Geometry: final body of the model. Coordinates: model frame, mm. A direction names the side the tool comes from. Give positions to 0.01 mm unless a question says otherwise; leave off trailing zeros. Loops run counter-clockwise (first coordinate to the right, second up) from the corner with the lowest first, then second, coordinate; pieces in that order, holes last. Notation, with made-up numbers: (-38.75, 1) -> (-29.75, 1) arc R13 cw to (-29.75, 16) -> close; hole circle Ø8 at (75, -9.75). An arc over 180 degrees is marked (long way). Answer in a Markdown table with one row per item. Add a question column.
1) Draft query along Y for faces 1 (the cylindrical face through (19.2, -37.5, 1)), 2 (the cylindrical face through (-29.97, 1.32, 26.65)), 3 (the cylindrical face through (6.466, -2.681, 0.986)), 4 (the flat face through (-1, -9, 0)). Return one class per face: +Y half, -Y half, draft (parallel to the pull), parting line (faces both ways), or undercut.
2) Section query D-D (x = -20). Return the cut outline in (y, z).
3) First-contact query: P1, Ø1.5, axis at x = 7, z = 37, coming from the -Y side; P2, Ø22.5, axis at x = 0, y = 0, coming from the +Z side; P3, Ø12, axis at x = -5, z = 34.5, coming from the +Y side; P4, Ø5.5, axis at x = -20, y = -36, coming from the -Z side. Flat tips, straight axial feed; report the tip coordinate or a pass-through.
4) Line query: line 1 (Y direction, x = 0, z = 0.95); line 2 (Y direction, x = -20, z = 1.6); line 3 (Z direction, x = 13, y = 18.5). Output: solid intervals per line, ascending. Write a range as from..to.
5) Access query for faces 5 (the cylindrical face through (25.865, -10.724, 26.65)), 6 (the cylindrical face through (-20.8, -37.5, 1)). Directions: +Z, -Z, +X, -X, +Y, -Y. A direction counts if a zero-diameter tool reaches every point of the face in a straight line with its end or side. Return the directions, or none.
6) Section query A-A (y = 0). Return the cut outline in (x, z), plus the area to 3 significant figures.
7) Section query B-B (y = -36). Return the cut outline in (x, z), plus the area to 3 significant figures.
```python
from build123d import *

# Parameters (mm, degrees)
SKETCH1_R                        = 45
SKETCH1_R_2                      = 7
GUARD_FLANGE_DEPTH               = 2
COUPLING_CONTACT_COVER_START     = 2
SKETCH2_R                        = 30
SKETCH2_R_2                      = 28
COUPLING_CONTACT_COVER_DEPTH     = 50
SKETCH3_R                        = 1.7
FOUR_M3_GUARD_FIXING_HOLES_DEPTH = 2.01


with BuildPart() as part:
    # Sketch1 → Guard_Flange (new body)
    with BuildSketch(Plane.XY):
        Circle(SKETCH1_R)
        Circle(SKETCH1_R_2, mode=Mode.SUBTRACT)
    extrude(amount=GUARD_FLANGE_DEPTH)

    # Sketch2 → Coupling_Contact_Cover (add)
    with BuildSketch(Plane.XY.offset(COUPLING_CONTACT_COVER_START)):
        Circle(SKETCH2_R)
        Circle(SKETCH2_R_2, mode=Mode.SUBTRACT)
    extrude(amount=COUPLING_CONTACT_COVER_DEPTH)

    # Sketch3 → Four_M3_Guard_Fixing_Holes (cut)
    with BuildSketch(Plane(origin=(0, 0, 0), x_dir=(-1, 0, 0), z_dir=(0, 0, -1))):
        with Locations((20, -36)):
            Circle(SKETCH3_R)
        with Locations((20, 36)):
            Circle(SKETCH3_R)
        with Locations((-20, -36)):
            Circle(SKETCH3_R)
        with Locations((-20, 36)):
            Circle(SKETCH3_R)
    extrude(amount=-FOUR_M3_GUARD_FIXING_HOLES_DEPTH, mode=Mode.SUBTRACT)


solid = part.part
```
Evaluation:
| question | item | result |
|---|---|---|
| 1 | face 1 | undercut |
| 1 | face 2 | parting line |
| 1 | face 3 | undercut |
| 1 | face 4 | draft |
| 2 | outline | (-40.31, 0) -> (-37.7, 0) -> (-37.7, 2) -> (-40.31, 2) -> close; (-34.3, 0) -> (34.3, 0) -> (34.3, 2) -> (22.36, 2) -> (22.36, 52) -> (19.6, 52) -> (19.6, 2) -> (-19.6, 2) -> (-19.6, 52) -> (-22.36, 52) -> (-22.36, 2) -> (-34.3, 2) -> close; (37.7, 0) -> (40.31, 0) -> (40.31, 2) -> (37.7, 2) -> close |
| 3 | P1 | y = -29.34 |
| 3 | P2 | z = 2 |
| 3 | P3 | y = 30 |
| 3 | P4 | z = 0 |
| 4 | line 1 | -45..-7, 7..45 |
| 4 | line 2 | -40.31..-37.7, -34.3..34.3, 37.7..40.31 |
| 4 | line 3 | 0..2 |
| 5 | face 5 | +Z |
| 5 | face 6 | +Z, -Z |
| 6 | outline | (-45, 0) -> (-7, 0) -> (-7, 2) -> (-28, 2) -> (-28, 52) -> (-30, 52) -> (-30, 2) -> (-45, 2) -> close; (7, 0) -> (45, 0) -> (45, 2) -> (30, 2) -> (30, 52) -> (28, 52) -> (28, 2) -> (7, 2) -> close |
| 6 | area | 352 mm² |
| 7 | outline | (-27, 0) -> (-21.7, 0) -> (-21.7, 2) -> (-27, 2) -> close; (-18.3, 0) -> (18.3, 0) -> (18.3, 2) -> (-18.3, 2) -> close; (21.7, 0) -> (27, 0) -> (27, 2) -> (21.7, 2) -> close |
| 7 | area | 94.4 mm² |
